```python
from build123d import *

# Parameters (mm, degrees)
F0_R           = 5.715
F1_DEPTH       = 101.6
F2_R           = 4.445
F3_DEPTH       = 99.06
F4_W           = 6.35
F4_H           = 8.89
F5_DEPTH       = 25.4
F8_DEPTH       = 8.89
F10_DEPTH      = 1.905
F10_DEPTH_BACK = 1.905


with BuildPart() as f1:
    # F0 (on Right) → F1 (new body)
    with BuildSketch(Plane.YZ):
        Circle(F0_R)
    extrude(amount=F1_DEPTH)

    # F2 (on face) → F3 (cut)
    with BuildSketch(Plane(origin=(0, 0, 0), x_dir=(0, -1, 0), z_dir=(-1, 0, 0))):
        Circle(F2_R)
    extrude(amount=-F3_DEPTH, mode=Mode.SUBTRACT)

    # F4 (on Top) → F5 (cut)
    with BuildSketch(Plane.XY):
        with Locations((95.885, 0)):
            Rectangle(F4_W, F4_H)
    extrude(amount=-F5_DEPTH, mode=Mode.SUBTRACT)

    # F7 (on offset) → F8 (join)
    with BuildSketch(Plane.YZ.offset(101.6)):
        with BuildLine():
            Line((6.985, 2.54), (5.119534, 2.54))
            ThreePointArc((5.119534, 2.54), (5.715, 0), (5.119534, -2.54))
            Line((5.119534, -2.54), (6.985, -2.54))
            Line((6.985, -2.54), (6.985, 2.54))
        make_face()
        with BuildLine():
            Line((-6.985, -2.54), (-5.119534, -2.54))
            ThreePointArc((-5.119534, -2.54), (-5.715, 0), (-5.119534, 2.54))
            Line((-5.119534, 2.54), (-6.985, 2.54))
            Line((-6.985, 2.54), (-6.985, -2.54))
        make_face()
    extrude(amount=-F8_DEPTH)

    # F9 (on Front) → F10 (join, two sides)
    with BuildSketch(Plane.XZ) as f10_sk:
        Polygon((102.235, 1.27), (103.124, 1.27), (103.124, -1.27), (101.6, -1.27), (101.6, -3.81), (104.14, -3.81), (104.14, 2.54), (102.235, 2.54), align=None)
    extrude(amount=F10_DEPTH)
    extrude(f10_sk.sketch, amount=-F10_DEPTH_BACK)


solid = f1.part
```
Build history of the part. All positions in model axes, mm. A direction names the side the tool comes from. Round coordinates to 2 decimals unless told otherwise and drop trailing zeros. Order: outer loops, then holes, each group sorted by start corner. A loop starts at its lowest first (then second) coordinate and runs counter-clockwise, first axis right, second up. Notation, with made-up numbers: (-14.5, 57) -> (17.5, 57) arc R23 cw to (17.5, 65) -> close; hole circle Ø3 at (-12, 35). An arc over 180 degrees is marked (long way). Answer in a Markdown table with one row per item.
1) Which spindle directions (+Z, -Z, +X, -X, +Y, -Y) get a long thin tool onto all of the face, cutting with end or side? Do faces 4 (the flat face through (99.06, 0, -1)), 5 (the flat face through (103, 0, 2.54)), 6 (the flat face through (97, 6, 2.54)), 7 (the flat face through (97, -6, 2.54)). Say none if no direction does.
Values:
| item | result |
|---|---|
| face 4 | -Z |
| face 5 | +Z, +X, +Y, -Y |
| face 6 | +Z, +X, -X, +Y |
| face 7 | +Z, +X, -X, -Y |
2) Band-saw the part on A-A on y = 0. Give the cut face in (x, z) (3 decimals).
Values:
| item | result |
|---|---|
| outline | (0, -5.715) -> (92.71, -5.715) -> (92.71, -4.445) -> (0, -4.445) -> close; (0, 4.445) -> (99.06, 4.445) -> (99.06, -5.715) -> (101.6, -5.715) -> (101.6, -3.81) -> (104.14, -3.81) -> (104.14, 2.54) -> (102.235, 2.54) -> (102.235, 1.27) -> (103.124, 1.27) -> (103.124, -1.27) -> (101.6, -1.27) -> (101.6, 5.715) -> (0, 5.715) -> close |
3) Wall check: L1, parallel to X at y = -1.75, z = 2.5 (3 decimals); L2, parallel to Z at x = 28.5, y = 0 (3 decimals). Give the ranges that are in metal, low to high.
Values:
| item | result |
|---|---|
| L1 | 99.06 to 101.6, 102.235 to 104.14 |
| L2 | -5.715 to -4.445, 4.445 to 5.715 |
4) Mould opens along Z. For faces 1 (the flat face through (96, -4.445, -2)), 2 (the cylindrical face through (48.837, 0.579, 4.407)), 3 (the flat face through (97, 6, -2.54)) say: released by +Z, released by -Z, zero draft, split by the parting line, or undercut.
Values:
| item | result |
|---|---|
| face 1 | zero draft |
| face 2 | undercut |
| face 3 | released by -Z |
5) Pin check, flat tips, straight feed: P1, Ø5, axis at y = -3, z = 1, coming from the -X side; P2, Ø3, axis at x = 36.5, z = 2.5, coming from the +Y side; P3, Ø0.6, axis at x = 99, y = -6.5, coming from the -Z side; P4, Ø1.7, axis at x = 102.5, y = -0.5, coming from the +Z side. Stop position of each tip, or through.
Values:
| item | result |
|---|---|
| P1 | x = 0 |
| P2 | y = 5.63 |
| P3 | z = -2.54 |
| P4 | z = 2.54 |
6) Band-saw the part on B-B on x = 87.5. Give the cut face in (y, z) (3 decimals), and give its area (3 significant figures).
Values:
| item | result |
|---|---|
| outline | circle Ø11.43 at (0, 0); hole circle Ø8.89 at (0, 0) |
| area | 40.5 mm2 |
